```python
from build123d import *

# Parameters (mm, degrees)
F0_W      = 304.8
F0_H      = 304.8
F0_W_2    = 292.1
F0_H_2    = 292.1
F1_DEPTH  = 152.4
F2_W      = 304.8
F2_H      = 304.8
F3_DEPTH  = 6.35
F5_D      = 0.0254
F5_DEPTH  = 12.7
F6_D      = 0.0254
F6_DEPTH  = 12.7
F8_D      = 0.0254
F8_DEPTH  = 12.7
F9_D      = 0.0254
F9_DEPTH  = 12.7
F12_D     = 0.0254
F12_DEPTH = 12.7
F13_D     = 0.0254
F13_DEPTH = 12.7
F14_D     = 0.0254
F14_DEPTH = 12.7
F15_D     = 0.0254
F15_DEPTH = 12.7
F16_D     = 0.0254
F16_DEPTH = 12.7
F17_D     = 0.0254
F17_DEPTH = 12.7


with BuildPart() as f1:
    # F0 (on Top) → F1 (new body, symmetric)
    with BuildSketch(Plane.XY):
        Rectangle(F0_W, F0_H)
        Rectangle(F0_W_2, F0_H_2, mode=Mode.SUBTRACT)
    extrude(amount=F1_DEPTH, both=True)

    # F2 (on face) → F3 (join)
    with BuildSketch(Plane.XY.offset(152.4)):
        Rectangle(F2_W, F2_H)
    extrude(amount=-F3_DEPTH)

    # F5
    with Locations(Plane(origin=(0, 152.4, 0), x_dir=(-1, 0, 0), z_dir=(0, 1, 0))):
        with Locations((38.1, 0)):
            Hole(F5_D / 2, depth=F5_DEPTH)

    # F6
    with Locations(Plane(origin=(0, 152.4, 0), x_dir=(-1, 0, 0), z_dir=(0, 1, 0))):
        with Locations((-106.68, -120.65)):
            Hole(F6_D / 2, depth=F6_DEPTH)

    # F8
    with Locations(Plane.XZ.offset(152.4)):
        with Locations((-106.68, -120.65)):
            Hole(F8_D / 2, depth=F8_DEPTH)

    # F9
    with Locations(Plane.XZ.offset(152.4)):
        with Locations((38.1, 0)):
            Hole(F9_D / 2, depth=F9_DEPTH)

    # F12
    with Locations(Plane.YZ.offset(152.4)):
        with Locations((-106.68, -120.65)):
            Hole(F12_D / 2, depth=F12_DEPTH)

    # F13
    with Locations(Plane.YZ.offset(152.4)):
        with Locations((76.2, 76.2)):
            Hole(F13_D / 2, depth=F13_DEPTH)

    # F14
    with Locations(Plane.YZ.offset(152.4)):
        with Locations((-120.65, 45.72)):
            Hole(F14_D / 2, depth=F14_DEPTH)

    # F15
    with Locations(Plane(origin=(-152.4, 0, 0), x_dir=(0, -1, 0), z_dir=(-1, 0, 0))):
        with Locations((-106.68, -120.65)):
            Hole(F15_D / 2, depth=F15_DEPTH)

    # F16
    with Locations(Plane(origin=(-152.4, 0, 0), x_dir=(0, -1, 0), z_dir=(-1, 0, 0))):
        with Locations((-120.65, 45.72)):
            Hole(F16_D / 2, depth=F16_DEPTH)

    # F17
    with Locations(Plane(origin=(-152.4, 0, 0), x_dir=(0, -1, 0), z_dir=(-1, 0, 0))):
        with Locations((76.2, 76.2)):
            Hole(F17_D / 2, depth=F17_DEPTH)


solid = f1.part
```
The listing builds one solid part. Answer for the finished solid, in the listing's coordinates (mm). A direction names the side the tool comes from. Give positions to 0.01 mm unless a question says otherwise; leave off trailing zeros. Order: outer loops, then holes, each group sorted by start corner. A loop starts at its lowest first (then second) coordinate and runs counter-clockwise, first axis right, second up. Notation, with made-up numbers: M -23,20.5 L -8,20.5 A15 ccw -8,28.5 Z; hole C 84,42 d9. An arc over 180 degrees is marked long. Put each result on its own line as item: value. Start each with the question number.
Item 1: The part is cut by section A-A, the plane z = 40. Determine the outline of the cut face in (x, y), and give its area (3 significant figures).
Item 2: For a pull along Y with two mould halves and no side action, classify faces 3 (the face through (-2, -152.4, 2)), 4 (the face through (-2, -146.05, -1)), 5 (the face through (-2, 152.4, 2)) as +Y half, -Y half, draft (parallel to the pull), parting line (faces both ways), or undercut.
Item 3: The part is cut by section B-B, the plane x = 89.5. Determine the outline of the cut face in (y, z), and give its area (3 significant figures).
Item 4: Which of the six approach directions +Z, -Z, +X, -X, +Y, -Y give full straight-line access (tool end or side, diameter ignored) to faces 1 (the face through (-2, 146.05, -1)), 2 (the face through (-2, 2, 152.4))?
Item 5: Find the intervals of material crossed by line 1 along Y through (x, z) = (105.5, -26); line 2 along Z through (x, y) = (-100, -38), in increasing order.
Item 6: A flat-ended cylindrical pin translates along its axis: P1, Ø6, axis at x = -54.5, y = 36.5, coming from the -Z side. Find the tip coordinate at first contact, or state that the pin passes through.
Answer key:
1. outline: M -152.4,-152.4 L 152.4,-152.4 L 152.4,152.4 L -152.4,152.4 Z; hole M -146.05,-146.05 L 146.05,-146.05 L 146.05,146.05 L -146.05,146.05 Z
1. area: 7,580 mm²
2. face 3: -Y half
2. face 4: undercut
2. face 5: +Y half
3. outline: M -152.4,-152.4 L -146.05,-152.4 L -146.05,146.05 L 146.05,146.05 L 146.05,-152.4 L 152.4,-152.4 L 152.4,152.4 L -152.4,152.4 Z
3. area: 5,730 mm²
4. face 1: -Z
4. face 2: +Z, +X, -X, +Y, -Y
5. line 1: y = -152.4 to -146.05, 146.05 to 152.4
5. line 2: z = 146.05 to 152.4
6. P1: stops at z = 146.05
